Read the model definition and answer for the solid it produces. Units are mm, in the model's axes. A direction names the side the tool comes from. Round coordinates to 2 decimals unless told otherwise and drop trailing zeros. Order: outer loops, then holes, each group sorted by start corner. A loop starts at its lowest first (then second) coordinate and runs counter-clockwise, first axis right, second up. Notation, with made-up numbers: (-27, 15) -> (9, 15) arc R16 ccw to (9, 42) -> close; hole circle Ø10 at (11.5, 20). An arc over 180 degrees is marked (long way). Use a Markdown table: item, result. Add a question column.
1. The mould has two halves that part along Y. Classify faces 5 (the face through (-52.113, -44.435, 2.958)), 6 (the face through (90, -30, 3)), 7 (the face through (120, 50, 3)): +Y half, -Y half, draft (parallel to the pull), parting line (faces both ways), or undercut.
2. Consider L1, parallel to Y at x = 134, z = 3 (3 decimals); L2, parallel to Y at x = 90, z = 2.5; L3, parallel to Y at x = 118, z = 5.75. Determine where each line is inside the solid, lowest interval first. Write a range as [from, to].
3. For faces 1 (the face through (0.801, -79.996, 2.958)), 2 (the face through (90, 30, 3)), 3 (the face through (99, -40, 3)), 4 (the face through (120, -50, 3)), determine the directions among +Z, -Z, +X, -X, +Y, -Y from which every point of the face is accessible in a straight line to the end or side of a thin tool.
4. Section C-C, the plane y = 76 is taken. Give the vertices of the cut face in (x, z).
5. Section B-B, the plane x = -55.5 is taken. Give the vertices of the cut face in (y, z).
6. Section A-A, the plane x = 0 is taken. Give the vertices of the cut face in (y, z).
7. Section D-D, the plane x = 50 is taken. Give the vertices of the cut face in (y, z), then the cut area to 3 significant figures.
8. Given pin 1 (1.5 mm diameter, centred on y = -56.5, z = 2.5, fed in from +X); pin 2 (3 mm diameter, centred on y = 38.5, z = 2.5, fed in from -X); pin 3 (2 mm diameter, centred on y = 24.5, z = 3, fed in from -X); pin 4 (2.5 mm diameter, centred on x = 114, y = 5.49, fed in from +Z), each flat-ended and moving along its own axis, determine where each tip first touches the part or whether it passes through.
```python
from build123d import *

# Parameters (mm, degrees)
SKETCH_1_R           = 87
SKETCH_1_R_2         = 1.55
EXTRUDE_1_DEPTH      = 6
SKETCH_2_R           = 1.55
CUT_EXTRUDE_1_DEPTH  = 40
SKETCH_3_W           = 100
SKETCH_3_H           = 60
EXTRUDE_2_DEPTH      = 6
CUT_EXTRUDE_2_DEPTH  = 40
SKETCH_5_R           = 58
SKETCH_5_R_2         = 52
EXTRUDE_3_DEPTH      = 6
CUT_EXTRUDE_3_DEPTH  = 70
FILLET_2_R           = 2
SKETCH_7_W           = 38
SKETCH_7_H           = 100
EXTRUDE_4_DEPTH      = 6
SKETCH_8_W           = 40
SKETCH_8_H           = 36
CUT_EXTRUDE_4_DEPTH  = 20
FILLET_3_R           = 2
SKETCH_9_R           = 1.525
CUT_EXTRUDE_5_DEPTH  = 80
SKETCH_10_R          = 1.525
CUT_EXTRUDE_6_DEPTH  = 80
SKETCH_11_W          = 25.06
SKETCH_11_H          = 3.06
CUT_EXTRUDE_7_DEPTH  = 30
SKETCH_12_R          = 1.505
CUT_EXTRUDE_8_DEPTH  = 60
SKETCH_13_W          = 4
SKETCH_13_H          = 100
EXTRUDE_5_DEPTH      = 6
SKETCH_14_R          = 1.525
CUT_EXTRUDE_9_DEPTH  = 6
SKETCH_15_W          = 32
SKETCH_15_H          = 31.510193749
SKETCH_15_H_2        = 34.459806251
CUT_EXTRUDE_10_DEPTH = 6
FILLET_4_R           = 2


with BuildPart() as part:
    # 草图1 → 凸台-拉伸1 (new body)
    with BuildSketch(Plane.XY):
        Circle(SKETCH_1_R)
        with Locations((24, 18)):
            Circle(SKETCH_1_R_2, mode=Mode.SUBTRACT)
        with Locations((-24, 18)):
            Circle(SKETCH_1_R_2, mode=Mode.SUBTRACT)
        with Locations((-24, -18)):
            Circle(SKETCH_1_R_2, mode=Mode.SUBTRACT)
        with Locations((24, -18)):
            Circle(SKETCH_1_R_2, mode=Mode.SUBTRACT)
    extrude(amount=EXTRUDE_1_DEPTH)

    # 草图2 → 切除-拉伸1 (cut)
    with BuildSketch(Plane.XY.offset(6)):
        with Locations((59.39696962, 59.39696962)):
            Circle(SKETCH_2_R)
        with Locations((59.39696962, -59.39696962)):
            Circle(SKETCH_2_R)
        with Locations((-59.39696962, -59.39696962)):
            Circle(SKETCH_2_R)
        with Locations((-59.39696962, 59.39696962)):
            Circle(SKETCH_2_R)
    extrude(amount=-CUT_EXTRUDE_1_DEPTH, mode=Mode.SUBTRACT)

    # 草图3 → 凸台-拉伸2 (add)
    with BuildSketch(Plane.XY.offset(6)):
        with Locations((87, 0)):
            Rectangle(SKETCH_3_W, SKETCH_3_H)
    extrude(amount=-EXTRUDE_2_DEPTH)

    # 草图4 → 切除-拉伸2 (cut)
    with BuildSketch(Plane(origin=(0, 0, 0), x_dir=(-1, 0, 0), z_dir=(0, 0, -1))):
        with BuildLine():
            Line((23.788509037, -23), (-23.788509037, -23))
            Line((-23.788509037, -23), (-53.929203709, -59.090109048))
            ThreePointArc((-53.929203709, -59.090109048), (0, -80), (53.929203709, -59.090109048))
            Line((53.929203709, -59.090109048), (23.788509037, -23))
        make_face()
        with BuildLine():
            Line((29, 16.759822751), (29, -16.759822751))
            Line((29, -16.759822751), (59.584985836, -53.38192075))
            ThreePointArc((59.584985836, -53.38192075), (74.722148212, -28.576223798), (80, 0))
            ThreePointArc((80, 0), (74.722148212, 28.576223798), (59.584985836, 53.38192075))
            Line((59.584985836, 53.38192075), (29, 16.759822751))
        make_face()
        with BuildLine():
            Line((-59.584985836, -53.38192075), (-29, -16.759822751))
            Line((-29, -16.759822751), (-29, 16.759822751))
            Line((-29, 16.759822751), (-59.584985836, 53.38192075))
            ThreePointArc((-59.584985836, 53.38192075), (-80, 0), (-59.584985836, -53.38192075))
        make_face()
        with BuildLine():
            Line((-53.929203709, 59.090109048), (-23.788509037, 23))
            Line((-23.788509037, 23), (23.788509037, 23))
            Line((23.788509037, 23), (53.929203709, 59.090109048))
            ThreePointArc((53.929203709, 59.090109048), (0, 80), (-53.929203709, 59.090109048))
        make_face()
    extrude(amount=-CUT_EXTRUDE_2_DEPTH, mode=Mode.SUBTRACT)

    # 草图5 → 凸台-拉伸3 (add)
    with BuildSketch(Plane(origin=(0, 0, 0), x_dir=(-1, 0, 0), z_dir=(0, 0, -1))):
        Circle(SKETCH_5_R)
        Circle(SKETCH_5_R_2, mode=Mode.SUBTRACT)
    extrude(amount=-EXTRUDE_3_DEPTH)

    # 草图6 → 切除-拉伸3 (cut)
    with BuildSketch(Plane(origin=(0, 0, 0), x_dir=(-1, 0, 0), z_dir=(0, 0, -1))):
        with BuildLine():
            Line((-45.276728704, 36.249383966), (-41.343228936, 31.539458162))
            Line((-41.343228936, 31.539458162), (-41.343228936, -31.539458162))
            Line((-41.343228936, -31.539458162), (-45.276728704, -36.249383966))
            ThreePointArc((-45.276728704, -36.249383966), (-58, 0), (-45.276728704, 36.249383966))
        make_face()
    extrude(amount=-CUT_EXTRUDE_3_DEPTH, mode=Mode.SUBTRACT)

    # 圆角2
    fillet_2_edges = [part.edges().sort_by_distance(p)[0] for p in [
        (-23.788509037, 23, 3),
        (23.788509037, 23, 3),
        (53.929203709, 59.090109048, 3),
        (53.929203709, -59.090109048, 3),
        (23.788509037, -23, 3),
        (-23.788509037, -23, 3),
        (-53.929203709, -59.090109048, 3),
        (-41.343228936, 31.539458162, 3),
        (-45.276728704, 36.249383966, 3),
        (39.808222335, -42.181814026, 3),
        (-39.808222335, 42.181814026, 3),
        (39.808222335, 42.181814026, 3),
        (-39.808222335, -42.181814026, 3),
        (35.954274067, -37.567142243, 3),
        (-35.954274067, -37.567142243, 3),
        (-35.954274067, 37.567142243, 3),
        (35.954274067, 37.567142243, 3),
        (-41.343228936, -31.539458162, 3),
        (-45.276728704, -36.249383966, 3),
        (-59.584985836, -53.38192075, 3),
        (-29, -16.759822751, 3),
        (-29, 16.759822751, 3),
        (-59.584985836, 53.38192075, 3),
        (59.584985836, 53.38192075, 3),
        (29, 16.759822751, 3),
        (29, -16.759822751, 3),
        (59.584985836, -53.38192075, 3),
        (-53.929203709, 59.090109048, 3),
    ]]
    fillet(fillet_2_edges, radius=FILLET_2_R)

    # 草图7 → 凸台-拉伸4 (add)
    with BuildSketch(Plane(origin=(0, 0, 0), x_dir=(-1, 0, 0), z_dir=(0, 0, -1))):
        with Locations((-118, 0)):
            Rectangle(SKETCH_7_W, SKETCH_7_H)
    extrude(amount=-EXTRUDE_4_DEPTH)

    # 草图8 → 切除-拉伸4 (cut, symmetric)
    with BuildSketch(Plane(origin=(0, 0, 0), x_dir=(-1, 0, 0), z_dir=(0, 0, -1))):
        Rectangle(SKETCH_8_W, SKETCH_8_H)
    extrude(amount=CUT_EXTRUDE_4_DEPTH, both=True, mode=Mode.SUBTRACT)

    # 圆角3
    fillet_3_edges = [part.edges().sort_by_distance(p)[0] for p in [
        (-20, 18, 3),
        (-20, -18, 3),
        (20, -18, 3),
        (20, 18, 3),
    ]]
    fillet(fillet_3_edges, radius=FILLET_3_R)

    # 草图9 → 切除-拉伸5 (cut)
    with BuildSketch(Plane(origin=(0, 0, 0), x_dir=(-1, 0, 0), z_dir=(0, 0, -1))):
        with Locations((-134, -43)):
            Circle(SKETCH_9_R)
        with Locations((-114, -43)):
            Circle(SKETCH_9_R)
        with Locations((-114, 43)):
            Circle(SKETCH_9_R)
        with Locations((-134, 43)):
            Circle(SKETCH_9_R)
    extrude(amount=-CUT_EXTRUDE_5_DEPTH, mode=Mode.SUBTRACT)

    # 草图10 → 切除-拉伸6 (cut)
    with BuildSketch(Plane.XY.offset(6)):
        with Locations((90, -17.118993381)):
            Circle(SKETCH_10_R)
        with Locations((90, 2.881006619)):
            Circle(SKETCH_10_R)
    extrude(amount=-CUT_EXTRUDE_6_DEPTH, mode=Mode.SUBTRACT)

    # 草图11 → 切除-拉伸7 (cut)
    with BuildSketch(Plane(origin=(0, 0, 0), x_dir=(-1, 0, 0), z_dir=(0, 0, -1))):
        with Locations((-117.5, 0.989806251)):
            Rectangle(SKETCH_11_W, SKETCH_11_H)
    extrude(amount=-CUT_EXTRUDE_7_DEPTH, mode=Mode.SUBTRACT)

    # 草图12 → 切除-拉伸8 (cut)
    with BuildSketch(Plane(origin=(0, 0, 0), x_dir=(-1, 0, 0), z_dir=(0, 0, -1))):
        with Locations((-128.525, 2.519806251)):
            Circle(SKETCH_12_R)
        with Locations((-128.525, -0.540193749)):
            Circle(SKETCH_12_R)
        with Locations((-106.475, 2.519806251)):
            Circle(SKETCH_12_R)
        with Locations((-106.475, -0.540193749)):
            Circle(SKETCH_12_R)
    extrude(amount=-CUT_EXTRUDE_8_DEPTH, mode=Mode.SUBTRACT)

    # 草图13 → 凸台-拉伸5 (add)
    with BuildSketch(Plane(origin=(0, 0, 0), x_dir=(-1, 0, 0), z_dir=(0, 0, -1))):
        with Locations((-139, 0)):
            Rectangle(SKETCH_13_W, SKETCH_13_H)
    extrude(amount=-EXTRUDE_5_DEPTH)

    # 草图14 → 切除-拉伸9 (cut)
    with BuildSketch(Plane(origin=(0, 0, 0), x_dir=(-1, 0, 0), z_dir=(0, 0, -1))):
        with Locations((-134, 5.489806251)):
            Circle(SKETCH_14_R)
        with Locations((-114, 5.489806251)):
            Circle(SKETCH_14_R)
    extrude(amount=-CUT_EXTRUDE_9_DEPTH, mode=Mode.SUBTRACT)

    # 草图15 → 切除-拉伸10 (cut)
    with BuildSketch(Plane.XY.offset(6)):
        with Locations((120, 24.244903126)):
            Rectangle(SKETCH_15_W, SKETCH_15_H)
        with Locations((120, -22.770096874)):
            Rectangle(SKETCH_15_W, SKETCH_15_H_2)
    extrude(amount=-CUT_EXTRUDE_10_DEPTH, mode=Mode.SUBTRACT)

    # 圆角4
    fillet_4_edges = [part.edges().sort_by_distance(p)[0] for p in [
        (99, 30, 3),
        (99, -30, 3),
        (81.663945533, 30, 3),
        (99, 50, 3),
        (99, -50, 3),
        (81.663945533, -30, 3),
        (141, 50, 3),
        (141, -50, 3),
        (136, 40, 3),
        (136, 8.489806251, 3),
        (104, 8.489806251, 3),
        (104, 40, 3),
        (136, -5.540193749, 3),
        (136, -40, 3),
        (104, -40, 3),
        (104, -5.540193749, 3),
    ]]
    fillet(fillet_4_edges, radius=FILLET_4_R)


solid = part.part
```
Verdict:
| question | item | result |
|---|---|---|
| 1 | face 5 | undercut |
| 1 | face 6 | -Y half |
| 1 | face 7 | +Y half |
| 2 | L1 | y = [-50, -44.525], [-41.475, -40], [-5.54, 3.965], [7.015, 8.49], [40, 41.475], [44.525, 50] |
| 2 | L2 | y = [-30, -18.64], [-15.59, 1.36], [4.41, 30] |
| 2 | L3 | y = [-50, -40], [-5.54, -0.54], [2.52, 8.49], [40, 50] |
| 3 | face 1 | +Z, -Z |
| 3 | face 2 | +Z, -Z, +Y |
| 3 | face 3 | +Z, -Z, -Y |
| 3 | face 4 | +Z, -Z, +X, -Y |
| 4 | outline | (-42.34, 0) -> (-24.98, 0) -> (-24.98, 6) -> (-42.34, 6) -> close; (24.98, 0) -> (42.34, 0) -> (42.34, 6) -> (24.98, 6) -> close |
| 5 | outline | (-67, 0) -> (-48.49, 0) -> (-48.49, 6) -> (-67, 6) -> close; (-16.84, 0) -> (16.84, 0) -> (16.84, 6) -> (-16.84, 6) -> close; (48.49, 0) -> (67, 0) -> (67, 6) -> (48.49, 6) -> close |
| 6 | outline | (-87, 0) -> (-80, 0) -> (-80, 6) -> (-87, 6) -> close; (-58, 0) -> (-52, 0) -> (-52, 6) -> (-58, 6) -> close; (-23, 0) -> (-18, 0) -> (-18, 6) -> (-23, 6) -> close; (18, 0) -> (23, 0) -> (23, 6) -> (18, 6) -> close; (52, 0) -> (58, 0) -> (58, 6) -> (52, 6) -> close; (80, 0) -> (87, 0) -> (87, 6) -> (80, 6) -> close |
| 7 | outline | (-71.2, 0) -> (-62.45, 0) -> (-62.45, 6) -> (-71.2, 6) -> close; (-54.39, 0) -> (-41.9, 0) -> (-41.9, 6) -> (-54.39, 6) -> close; (41.9, 0) -> (54.39, 0) -> (54.39, 6) -> (41.9, 6) -> close; (62.45, 0) -> (71.2, 0) -> (71.2, 6) -> (62.45, 6) -> close |
| 7 | area | 255 mm2 |
| 8 | pin 1 | stops at x = 66.79 |
| 8 | pin 2 | stops at x = -78.74 |
| 8 | pin 3 | stops at x = -83.77 |
| 8 | pin 4 | passes through |
